Read the model definition and answer for the solid it produces. Units are mm, in the model's axes. A direction names the side the tool comes from. Coordinates: 2 decimals unless noted, no trailing zeros. Order: outer loops, then holes, each group sorted by start corner. A loop starts at its lowest first (then second) coordinate and runs counter-clockwise, first axis right, second up. Notation, with made-up numbers: (82.5, 74) - (132.5, 74) arc R21 cw to (132.5, 111) - close; hole circle Ø8 at (1.25, 64.25). An arc over 180 degrees is marked (long way). Use one line per item in the form item = value.
Autodesk Inventor part; units mm, degrees
ref_plane "YZ Plane" through (0, 0, 0) normal (1, 0, 0) x (0, 1, 0)
ref_plane "XZ Plane" through (0, 0, 0) normal (0, 1, 0) x (-1, 0, 0)
ref_plane "XY Plane" through (0, 0, 0) normal (0, 0, 1) x (1, 0, 0)
sketch "Sketch1" plane through (0, 0, 0) normal (0, 0, 1) x (1, 0, 0)
  line L0 (-490, 68) -> (490, 68)
  line L1 (490, 68) -> (490, 0)
  line L2 (490, 0) -> (-490, 0)
  line L3 (-490, 0) -> (-490, 68)
  point P0 (0, 0)
  point P1 (0, 0)
  dimension "d0" = 980
  dimension "d1" = 68
extrude "Plate1" add sketch "Sketch1" along normal blind 2
sketch "Sketch2" plane through (490, 2, 0) normal (0, -1, 0) x (1, 0, 0)
  line L0 (-980, 0) -> (0, 0)
  line L1 (0, 0) -> (0, 20)
  line L2 (0, 20) -> (-980, 20)
  line L3 (-980, 20) -> (-980, 0)
edge flange "Flange1" height 20 angle 90 thickness 2 bend radius 2.75 thickness toward (0, -1, 0) relief round relief width 2 relief depth 1 edges at (0, 0, 2) wall of the first edge with corners at (-490, 2, 0) (490, 2, 0) (490, 2, 20) (-490, 2, 20)
bend "Bend1"
corner "Corner1"
sketch "Sketch5" plane through (0, 0, 0) normal (0, 0, -1) x (-1, 0, 0)
  line L0 (490, 68) -> (-490, 68)
  line L1 (490, 0) -> (-490, 0)
  circle A0 centre (0, 68) radius 35
  line L2 (243.95, 68) -> (246.05, 68)
  line L3 (246.05, 68) -> (246.05, 27)
  line L4 (246.05, 27) -> (243.95, 27)
  line L5 (243.95, 27) -> (243.95, 68)
  line L6 (-243.95, 68) -> (-246.05, 68)
  line L7 (-246.05, 68) -> (-246.05, 27)
  line L8 (-246.05, 27) -> (-243.95, 27)
  line L9 (-243.95, 27) -> (-243.95, 68)
  line L10 (0, 68) -> (0, 0) construction
  line L11 (0, 68) -> (0, 0)
  line L12 (490, 68) -> (490, 4.75)
  line L13 (490, 0) -> (490, 4.75)
  line L14 (-490, 4.75) -> (-490, 68)
  line L15 (-490, 4.75) -> (-490, 0)
  point P0 (0, 0)
  point P1 (245, 27)
  point P2 (-245, 27)
  point P3 (-35, 68)
  point P4 (35, 68)
  dimension "d45" = 70
  dimension "d48" = 2.1
  dimension "d49" = 490
  dimension "d51" = 27
  dimension "d52" = 41
extrude "Extrusion1" cut sketch "Sketch5" against normal through all contours L12 L13 L1 L11 A0 L0 L5 L4 L3 | L3 L4 L5 L0 | A0 L11 L0 | L9 L8 L7 L0 picked at (23.0408, 65.4039)
sketch "Sketch9" plane through (0, 0, 2) normal (0, 0, 1) x (1, 0, 0)
  line L0 (485.6141, 29.596) -> (485.6141, 17.596) construction
  line L1 (485.6141, 17.596) -> (285.6141, 17.596) construction
  line L2 (285.6141, 17.596) -> (285.6141, 29.596) construction
  line L3 (285.6141, 29.596) -> (485.6141, 29.596) construction
  line L4 (-490, 68) -> (490, 68)
  point P0 (0, 0)
  point P1 (1.05, 68)
  dimension "d40" = 200
  dimension "d41" = 12
mark "Mark2"
equation "\"d1\" = СПИНА_Стрингер_2_высота"
equation "\"d2\" = Thickness"
equation "\"d3\" = BendReliefWidth"
equation "\"d4\" = BendReliefDepth"
equation "\"d5\" = MinimumRemnant"
equation "\"d6\" = TransitionRadius"
equation "\"d9\" = BendRadius"
equation "\"d10\" = CornerReliefSize"
equation "\"d11\" = GapSize"
equation "\"d12\" = JacobiRadiusSize"
equation "\"BendReliefWidth\" = Thickness"
equation "\"BendReliefDepth\" = 0.5 * Thickness"
equation "\"CornerReliefSize\" = 4 * Thickness"
equation "\"MinimumRemnant\" = 2 * Thickness"
equation "\"TransitionRadius\" = BendRadius"
equation "\"JacobiRadiusSize\" = BendRadius"
equation "\"GapSize\" = Thickness"
properties part number "MSC 207 STRINGER BACK ^^" material "Stainless Steel"
(1) Section C-C, the plane z = 13 is taken. Write down the section's boundary in (x, y), then the cut area to 3 significant figures.
Answer list:
outline = (0, 0) - (490, 0) - (490, 2) - (0, 2) - close
area = 980 mm2
(2) Section B-B, the plane x = 90.5 is taken. Write down the section's boundary in (y, z).
Answer list:
outline = (0, 4.75) arc R4.75 ccw to (4.75, 0) - (68, 0) - (68, 2) - (4.75, 2) arc R2.75 cw to (2, 4.75) - (2, 20) - (0, 20) - close
(3) Which of the six approach directions +Z, -Z, +X, -X, +Y, -Y give full straight-line access (tool end or side, diameter ignored) to faces 1 (the flat face through (242, 37, 0)), 2 (the flat face through (248, 2, 12))?
Answer list:
face_1 = -Z, +X, -X, +Y, -Y
face_2 = +Z, +X, -X, +Y
(4) A straight line is drawn through the part: L1, parallel to Z at x = 198, y = 61. Find the intervals that lie inside material, in ascending order.
Answer list:
L1 = 0 to 2
(5) Given pin 1 Ø8 at (x, y) = (142, 33.5) entering from +Z, flat-ended and moving along its own axis, determine where the tip first touches the part or whether it passes through.
Answer list:
pin_1 = 2
(6) Section A-A, the plane y = 55 is taken. Write down the section's boundary in (x, z).
Answer list:
outline = (0, 0) - (243.95, 0) - (243.95, 2) - (0, 2) - close; (246.05, 0) - (490, 0) - (490, 2) - (246.05, 2) - close
